from build123d import *

# Parameters (mm, degrees)
F1_DEPTH  = 3.9624
F2_R      = 23.0251
F3_DEPTH  = 7.9248
F5_DEPTH  = 2.9972
F6_R      = 6.35
F6_R_2    = 3.453465
F6_R_3    = 3.458119
F7_DEPTH  = 8.7122
F8_R      = 6.35
F9_DEPTH  = 23.5976
F10_R     = 3.175
F11_DEPTH = 14.8854


with BuildPart() as f1:
    # F0 (on Top) → F1 (new body)
    with BuildSketch(Plane.XY):
        with BuildLine():
            Line((-8.962085, -25.2095), (0, -25.2095))
            Line((0, -25.2095), (10.198205, -25.2095))
            ThreePointArc((10.198205, -25.2095), (12.737725, -27.767632), (11.69605, -31.218445))
            ThreePointArc((11.69605, -31.218445), (-0.134135, 33.33723), (-11.444457, -31.311552))
            ThreePointArc((-11.444457, -31.311552), (-12.615628, -27.667498), (-9.681515, -25.2095))
            Line((-9.681515, -25.2095), (-8.962085, -25.2095))
        make_face()
    extrude(amount=F1_DEPTH)

    # F2 (on face) → F3 (join)
    with BuildSketch(Plane.XY.offset(3.9624)):
        Circle(F2_R)
    extrude(amount=F3_DEPTH)

    # F4 (on face) → F5 (join)
    with BuildSketch(Plane.XY.offset(11.8872)):
        with BuildLine():
            Line((-24.286461, -22.84014), (24.286461, -22.84014))
            ThreePointArc((24.286461, -22.84014), (0, 33.339229), (-24.286461, -22.84014))
        make_face()
    extrude(amount=F5_DEPTH)

    # F6 (on face) → F7 (join)
    with BuildSketch(Plane.XY.offset(14.8844)):
        Circle(F6_R)
        with BuildLine():
            Line((8.7376, -7.221702), (21.298547, 6.35))
            ThreePointArc((21.298547, 6.35), (0, 22.225), (-21.298547, 6.35))
            Line((-21.298547, 6.35), (-8.7376, -7.221702))
            Line((-8.7376, -7.221702), (-8.7376, -11.966851))
            ThreePointArc((-8.7376, -11.966851), (-12.057279, -15.876777), (-16.453895, -13.23527))
            Line((-16.453895, -13.23527), (-17.271447, -13.987414))
            ThreePointArc((-17.271447, -13.987414), (-0.024306, -22.224987), (17.240811, -14.025158))
            Line((17.240811, -14.025158), (16.397809, -13.390516))
            ThreePointArc((16.397809, -13.390516), (11.975978, -15.862542), (8.7376, -11.966851))
            Line((8.7376, -11.966851), (8.7376, -7.221702))
        make_face()
        with Locations((0, -16.6624)):
            Circle(F6_R_2, mode=Mode.SUBTRACT)
        Circle(F6_R, mode=Mode.SUBTRACT)
        with Locations((0, 16.6624)):
            Circle(F6_R_3, mode=Mode.SUBTRACT)
    extrude(amount=F7_DEPTH)

    # F8 (on face) → F9 (cut, through all)
    with BuildSketch(Plane.XY.offset(23.5966)):
        Circle(F8_R)
    extrude(amount=-F9_DEPTH, mode=Mode.SUBTRACT)

    # F10 (on face) → F11 (cut, through all)
    with BuildSketch(Plane.XY.offset(14.8844)):
        with Locations((-12.7, -11.966851)):
            Circle(F10_R)
        with Locations((12.7, -11.966851)):
            Circle(F10_R)
    extrude(amount=-F11_DEPTH, mode=Mode.SUBTRACT)


solid = f1.part
Work out the finished part from the listing and answer in its coordinate system (mm). A direction names the side the tool comes from. Round coordinates to 2 decimals unless told otherwise and drop trailing zeros. Write each loop counter-clockwise with the first axis right and the second up, starting at its lowest first coordinate (ties: lowest second). Pieces come first, ordered by that corner, then holes.
1) Given pin 1 Ø3 at (y, z) = (-15, 16.5) entering from -X; pin 2 Ø1 at (x, z) = (21, 4.5) entering from +Y; pin 3 Ø4 at (x, y) = (-12.7, -11.97) entering from +Z; pin 4 Ø2 at (x, z) = (-1.5, 2) entering from -Y, each flat-ended and moving along its own axis, determine where each tip first touches the part or whether it passes through.
2) The mould has two halves that part along Z. Classify faces 4 (the flat face through (4.4, 5.3, 23.597)), 5 (the flat face through (0, 9, 0)), 6 (the cylindrical face through (12.725, -27.716, 1.953)), 7 (the cylindrical face through (-4.991, -22.478, 7.869)): pulls with the +Z half, pulls with the -Z half, needs draft (parallel to the pull), parting line crosses it, or undercut.
3) A cutting plane is placed at B-B (y = 24). Give the vertices of the cut face in (x, z), plus the area to 3 significant figures.
4) Straight lines are drawn through the part: line 1 (Z direction, x = 29.5, y = -5.5); line 2 (X direction, y = -7.5, z = 20.5); line 3 (Y direction, x = 12.7, z = 11). For each, find the intervals that lie inside material, in ascending order.
5) A tool of negligible diameter and unlimited length cuts with its end or side. For faces 1 (the flat face through (-15, -1, 14.884)), 2 (the flat face through (8.738, -10, 19)), 3 (the cylindrical face through (-12.63, -27.72, 1.95)), from which of +Z, -Z, +X, -X, +Y, -Y can it reach the whole face along a straight path? Write none if from no direction.
6) A cutting plane is placed at D-D (y = 12). Give the vertices of the cut face in (x, z), plus the area to 3 significant figures.
7) A cutting plane is placed at C-C (z = 2.5). Give the number of separate pieces and of enclosed holes in the cut face, plus the area to 3 significant figures.
Completed:
1. pin 1: stops at x = -17.27
1. pin 2: stops at y = 10.48
1. pin 3: passes through
1. pin 4: stops at y = -25.21
2. face 4: pulls with the +Z half
2. face 5: pulls with the -Z half
2. face 6: needs draft
2. face 7: undercut
3. outline: (-23.14, 0) - (23.14, 0) - (23.14, 3.96) - (-23.14, 3.96) - close; (-23.14, 11.89) - (23.14, 11.89) - (23.14, 14.88) - (-23.14, 14.88) - close
3. area: 322 mm2
4. line 1: z = 0 to 3.96, 11.89 to 14.88
4. line 2: x = -8.74 to 8.74
4. line 3: y = -19.21 to -15.14, -8.79 to 19.21
5. face 1: +Z
5. face 2: +Z, +X
5. face 3: +Z, -Z
6. outline: (-31.1, 0) - (31.1, 0) - (31.1, 3.96) - (19.65, 3.96) - (19.65, 11.89) - (31.1, 11.89) - (31.1, 14.88) - (18.71, 14.88) - (18.71, 23.6) - (-18.71, 23.6) - (-18.71, 14.88) - (-31.1, 14.88) - (-31.1, 11.89) - (-19.65, 11.89) - (-19.65, 3.96) - (-31.1, 3.96) - close
6. area: 1,070 mm2
7. separate pieces: 1
7. enclosed holes: 3
7. area: 3,120 mm2
